from build123d import *

# Parameters (mm, degrees)
F0_W     = 69.85
F0_H     = 386.08
F0_W_2   = 25.4
F0_H_2   = 12.7
F0_H_3   = 64.6534590532
F1_DEPTH = 3.175


# Not quite as in the source:
# - the dataset's text gives a spline's control points without its knots; the knots are read off the source's solid


with BuildPart() as f1:
    # F0 (on Top) → F1 (new body)
    with BuildSketch(Plane.XY):
        with Locations((34.925, 257.6934590532)):
            Rectangle(F0_W, F0_H)
        with Locations((34.925, 337.7034590532)):
            Rectangle(F0_W_2, F0_H_2, mode=Mode.SUBTRACT)
        with BuildLine():
            Line((0, 0), (0, 64.6534590532))
            add(Edge.make_bspline(
                [(0, 64.6534590532), (0, 203.2), (-44.45, 203.2)],
                knots=[4.7123889804, 4.7123889804, 4.7123889804, 6.2831853072, 6.2831853072, 6.2831853072], degree=2, weights=[1, 0.7071067812, 1]))
            add(Edge.make_bspline(
                [(-44.45, 203.2), (-83.9884760445, 203.2), (-92.075, 92.9894)],
                knots=[0, 0, 0, 1.3648200427, 1.3648200427, 1.3648200427], degree=2, weights=[1, 0.7760550574, 1]))
            ThreePointArc((-92.075, 92.9894), (-120.4661612059, 50.3219990464), (-130.175, 0))
            Line((-130.175, 0), (0, 0))
        make_face()
        with Locations((34.925, 32.3267295266)):
            Rectangle(F0_W, F0_H_3)
        with BuildLine():
            add(Edge.make_bspline(
                [(114.3, 203.2), (116.5605862503, 203.2), (121.9530728583, 202.3331388879), (130.4947147155, 197.5987791483), (141.4933741705, 183.4269013443), (152.7385562531, 156.2534255189), (158.9074917941, 129.7692462355), (161.3044412153, 110.6229696373), (161.8811367628, 98.626656943), (161.925, 92.9830765781)],
                knots=[0.5267526841, 0.5267526841, 0.5267526841, 0.5267526841, 0.5267526841, 0.5267526841, 0.6, 0.7, 0.8, 0.9, 0.9934494331, 0.9934494331, 0.9934494331, 0.9934494331, 0.9934494331, 0.9934494331], degree=5))
            add(Edge.make_bspline(
                [(114.3, 203.2), (69.85, 203.2), (69.85, 64.6534590532)],
                knots=[0, 0, 0, 1.5707963268, 1.5707963268, 1.5707963268], degree=2, weights=[1, 0.7071067812, 1]))
            Line((69.85, 64.6534590532), (69.85, 0))
            Line((69.85, 0), (200.025, 0))
            ThreePointArc((200.025, 0), (190.3149490033, 50.3186009129), (161.925, 92.9830765781))
        make_face()
    extrude(amount=F1_DEPTH)


solid = f1.part
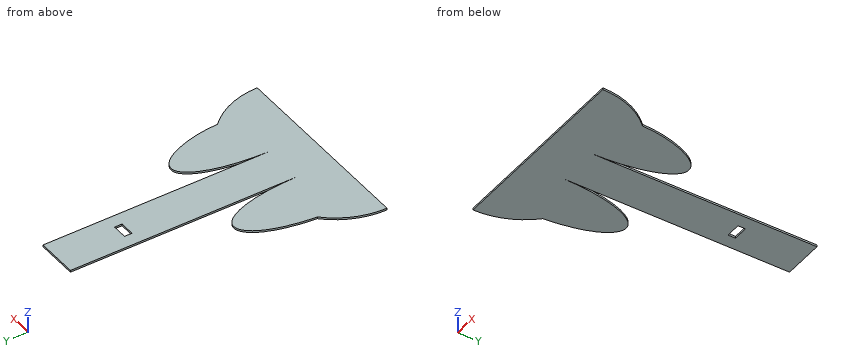
Could you check a few things on this model? Use its own coordinates, in mm. Give positions to 0.01 mm unless a question says otherwise; leave off trailing zeros. Order: outer loops, then holes, each group sorted by start corner. A loop starts at its lowest first (then second) coordinate and runs counter-clockwise, first axis right, second up. Notation, with made-up numbers: (15, -10) -> (44, -10) arc R10 ccw to (44, 7) -> close; hole circle Ø9 at (-29.5, 56). An arc over 180 degrees is marked (long way). Answer in a Markdown table with one row per item. Add a question column.
Item 1: I'm going to push flat-ended pins straight in: P1, Ø1, axis at y = 348, z = 2, coming from the -X side; P2, Ø1, axis at y = 51, z = 1.5, coming from the -X side. Where does each tip first touch, or does it pass through?
Item 2: Imagine slicing it at B-B (y = 75.5). Count the separate pieces of the cut face and the enclosed holes in it, and give its area (3 significant figures).
Item 3: Please list where these lines run through material, in increasing order: probe 1 along X at (y, z) = (334.5, 3) (3 decimals); probe 2 along Y at (x, z) = (36, 0.6); probe 3 along X at (y, z) = (93.5, 0.8).
Item 4: Imagine slicing it at A-A (y = 405). List the corners of the cut face in (x, z) for me (3 decimals), and give its area (3 significant figures).
Result:
| question | item | result |
|---|---|---|
| 1 | P1 | x = 0 |
| 1 | P2 | x = -120.39 |
| 2 | separate pieces | 3 |
| 2 | enclosed holes | 0 |
| 2 | area | 899 mm2 |
| 3 | probe 1 | 0 to 22.225, 47.625 to 69.85 |
| 3 | probe 2 | 0 to 331.35, 344.05 to 450.73 |
| 3 | probe 3 | -92.04 to -0.97, 0 to 69.85, 70.82 to 161.92 |
| 4 | outline | (0, 0) -> (69.85, 0) -> (69.85, 3.175) -> (0, 3.175) -> close |
| 4 | area | 222 mm2 |
